from build123d import *

# Parameters (mm, degrees)
F1_DEPTH = 3
F2_SIZE  = 3
F3_W     = 3.2
F3_H     = 80.2
F4_DEPTH = 3.001
F5_W     = 24.2
F5_H     = 3.2
F6_DEPTH = 3.001
F7_W     = 24.2
F7_H     = 3.2
F8_DEPTH = 3.001


# Not quite as in the source:
# - a pattern or mirror of a feature is missing from the dataset's text; its kind, count and spacing are read off the source's solid


with BuildPart() as f1:
    # F0 (on Top) → F1 (new body)
    with BuildSketch(Plane.XY):
        Polygon((117, 40), (117, 117), (40, 117), (40, 120), (-40, 120), (-40, 117), (-117, 117), (-117, 40), (-120, 40), (-120, -40), (-117, -40), (-117, -117), (-40, -117), (-40, -120), (40, -120), (40, -117), (117, -117), (117, -40), (120, -40), (120, 40), align=None)
    extrude(amount=F1_DEPTH)

    # F2
    f2_edges = [f1.edges().sort_by_distance(p)[0] for p in [
        (117, -117, 1.5),
        (-117, 117, 1.5),
        (117, 117, 1.5),
        (-117, -117, 1.5),
    ]]
    chamfer(f2_edges, length=F2_SIZE)

    # F3 (on face) → F4 (cut, through all)
    with BuildSketch(Plane.XY.offset(3)):
        with Locations((-39.5, 0)):
            Rectangle(F3_W, F3_H)
    f4 = extrude(amount=-F4_DEPTH, mode=Mode.SUBTRACT)

    # F4_copies: F4 across plane
    add(f4.mirror(Plane(origin=(0, 0, 0), x_dir=(0, 0, 1), z_dir=(1, 0, 0))), mode=Mode.SUBTRACT)

    # F5 (on face) → F6 (cut, through all)
    with BuildSketch(Plane.XY.offset(3)):
        with Locations((-79, 39.5)):
            Rectangle(F5_W, F5_H)
        with Locations((-79, -39.5)):
            Rectangle(F5_W, F5_H)
    f6 = extrude(amount=-F6_DEPTH, mode=Mode.SUBTRACT)

    # F6_copies: F6 across plane
    add(f6.mirror(Plane(origin=(0, 0, 0), x_dir=(0, 0, 1), z_dir=(1, 0, 0))), mode=Mode.SUBTRACT)

    # F7 (on face) → F8 (cut, through all)
    with BuildSketch(Plane.XY.offset(3)):
        with Locations((0, 39.5)):
            Rectangle(F7_W, F7_H)
        with Locations((0, -39.5)):
            Rectangle(F7_W, F7_H)
    extrude(amount=-F8_DEPTH, mode=Mode.SUBTRACT)


solid = f1.part
Read the model definition and answer for the solid it produces. Units are mm, in the model's axes. Give positions to 0.01 mm unless a question says otherwise; leave off trailing zeros. Write each loop counter-clockwise with the first axis right and the second up, starting at its lowest first coordinate (ties: lowest second). Pieces come first, ordered by that corner, then holes. Notation, with made-up numbers: (7, 40.5) -> (14, 40.5) arc R22 cw to (14, 55.5) -> close; hole circle Ø2 at (76, 24.5). An arc over 180 degrees is marked (long way). Answer as a JSON object with one key per item and string values. Group by question number.
1) Find section B-B (x = -80.5). Write down the section's boundary in (y, z).
2) Find section C-C (z = 1.85). Count the separate pieces of the cut face and the enclosed holes in it, and give its area (3 significant figures).
3) Consider L1, parallel to Y at x = -90, z = 2.1; L2, parallel to Y at x = -6.5, z = 1.05. Determine where each line is inside the solid, lowest interval first. Write a range as from..to.
4) Find section A-A (y = -17). Write down the section's boundary in (x, z), and give its area (3 significant figures).
5) Find section D-D (y = -57). Write down the section's boundary in (x, z).
6) Each of these flat-tipped pins is pushed along its axis until it touches: P1, Ø0.9, axis at x = 77.5, z = 2, coming from the -Y side; P2, Ø1.5, axis at y = -69.5, z = 2, coming from the -X side; P3, Ø0.9, axis at x = -75, z = 1, coming from the +Y side. Where does it stop, or does it pass through?
Values follow:
{
 "1": {"outline": "(-117, 0) -> (-41.1, 0) -> (-41.1, 3) -> (-117, 3) -> close; (-37.9, 0) -> (37.9, 0) -> (37.9, 3) -> (-37.9, 3) -> close; (41.1, 0) -> (117, 0) -> (117, 3) -> (41.1, 3) -> close"},
 "2": {"separate pieces": "1", "enclosed holes": "8", "area": "54,700 mm2"},
 "3": {"L1": "y = -117..-41.1, -37.9..37.9, 41.1..117", "L2": "y = -120..-41.1, -37.9..37.9, 41.1..120"},
 "4": {"outline": "(-120, 0) -> (-41.1, 0) -> (-41.1, 3) -> (-120, 3) -> close; (-37.9, 0) -> (37.9, 0) -> (37.9, 3) -> (-37.9, 3) -> close; (41.1, 0) -> (120, 0) -> (120, 3) -> (41.1, 3) -> close", "area": "701 mm2"},
 "5": {"outline": "(-117, 0) -> (117, 0) -> (117, 3) -> (-117, 3) -> close"},
 "6": {"P1": "stops at y = -117", "P2": "stops at x = -117", "P3": "stops at y = 117"}
}
